CAD build for the part. Positions are in the model's coordinates, mm. A direction names the side the tool comes from. Give positions to 0.01 mm unless a question says otherwise; leave off trailing zeros. Loops run counter-clockwise (first coordinate to the right, second up) from the corner with the lowest first, then second, coordinate; pieces in that order, holes last. Notation, with made-up numbers: M 73.5,-25 L 79.5,-25 A27 ccw 79.5,-4 Z; hole C -32,-25 d6. An arc over 180 degrees is marked long. Answer as CSV lines item,"result".
```python
from build123d import *

# Parameters (mm, degrees)
BOSS_EXTRU_1_DEPTH = 2
CONG_1_R           = 2


with BuildPart() as part:
    # Esquisse1 → Boss.-Extru.1 (new body)
    with BuildSketch(Plane(origin=(0, 0, 0), x_dir=(0, 0, -1), z_dir=(1, 0, 0))):
        Polygon((-20.500365221, -12.705219678), (-15.500365221, -12.705219678), (-15.500365221, -15.705219678), (-7.500365221, -15.705219678), (-7.500365221, -12.705219678), (-0.500365221, -12.705219678), (3.6407395, 2.749593542), (0.742962022, 3.526050678), (1.778238202, 7.389753983), (-3.051390929, 8.683849208), (-7.442828702, -7.705219678), (-20.500365221, -7.705219678), align=None)
    extrude(amount=BOSS_EXTRU_1_DEPTH)

    # Congé1
    cong_1_edges = [part.edges().sort_by_distance(p)[0] for p in [
        (1, -7.705219678, 20.500365221),
        (1, -7.705219678, 7.442828702),
        (1, 8.683849208, 3.051390929),
    ]]
    fillet(cong_1_edges, radius=CONG_1_R)


solid = part.part
```
Q1. Which spindle directions (+Z, -Z, +X, -X, +Y, -Y) get a long thin tool onto all of the face, cutting with end or side? Do faces 5 (the flat face through (0.986, 7.773, -0.35)), 6 (the flat face through (1, -14, 15.5)), 7 (the flat face through (1, -14, 7.5)), 8 (the cylindrical face through (1.014, 7.977, 2.618)), 9 (the flat face through (1, -7.705, 14)). Say none if no direction does.
Solution:
face 5,"-Z, +X, -X, +Y"
face 6,"+Z, +X, -X, -Y"
face 7,"-Z, +X, -X, -Y"
face 8,"+X, -X, +Y"
face 9,"+Z, +X, -X, +Y"
Q2. Pin check, flat tips, straight feed: P1, Ø1, axis at x = 1, z = 18, coming from the -Y side; P2, Ø0.6, axis at x = 1, y = -14, coming from the -Z side; P3, Ø1, axis at x = 1.5, y = 0, coming from the +Z side. Stop position of each tip, or through.
Solution:
P1,"stops at y = -12.71"
P2,"stops at z = 7.5"
P3,"stops at z = 5.51"
Q3. Cut at B-B (z = 18). Write the cut outline in (x, y).
Solution:
outline,"M 0,-12.71 L 2,-12.71 L 2,-7.71 L 0,-7.71 Z"
Q4. Cut at C-C (y = -13.75). Write the cut outline in (x, z), and give its area (3 significant figures).
Solution:
outline,"M 0,7.5 L 2,7.5 L 2,15.5 L 0,15.5 Z"
area,"16.0 mm²"
Q5. Wall check: line 1 (Y direction, x = 1.6, z = 17.5); line 2 (Y direction, x = 0.45, z = 9.5); line 3 (Z direction, x = 1.65, y = -13.75). Give the ranges that are in metal, low to high. Write a range as [from, to].
Solution:
line 1,"y = [-12.71, -7.71]"
line 2,"y = [-15.71, -7.71]"
line 3,"z = [7.5, 15.5]"
Q6. Cut at A-A (x = 1.4). Write the cut outline in (y, z).
Solution:
outline,"M -15.71,7.5 L -12.71,7.5 L -12.71,0.5 L 2.75,-3.64 L 3.53,-0.74 L 7.39,-1.78 L 8.17,1.12 A2 ccw 6.75,3.57 L -6.22,7.05 A2 cw -7.71,8.98 L -7.71,18.5 A2 ccw -9.71,20.5 L -12.71,20.5 L -12.71,15.5 L -15.71,15.5 Z"
Q7. Mould opens along Y. For faces 1 (the flat face through (0.986, 5.431, -1.253)), 2 (the flat face through (1, -12.705, 4)), 3 (the flat face through (2, -6, 6)), 4 (the flat face through (0.986, 3.132, -2.212)) say: released by +Y, released by -Y, zero draft, split by the parting line, or undercut.
Solution:
face 1,"undercut"
face 2,"released by -Y"
face 3,"zero draft"
face 4,"undercut"
